from build123d import *

# Parameters (mm, degrees)
SKETCH_1_W          = 100
SKETCH_1_H          = 80
SKETCH_1_R          = 1.5
SKETCH_1_R_2        = 2.5
EXTRUDE_1_DEPTH     = 3
SKETCH_2_R          = 1.5
CUT_EXTRUDE_1_DEPTH = 10
SKETCH_3_R          = 2
CUT_EXTRUDE_2_DEPTH = 65.101482042


with BuildPart() as part:
    # 草图1 → 凸台-拉伸1 (new body)
    with BuildSketch(Plane.XY):
        Rectangle(SKETCH_1_W, SKETCH_1_H)
        with Locations((0, 14)):
            Circle(SKETCH_1_R, mode=Mode.SUBTRACT)
        with Locations((12.124355653, 7)):
            Circle(SKETCH_1_R, mode=Mode.SUBTRACT)
        with Locations((12.124355653, -7)):
            Circle(SKETCH_1_R, mode=Mode.SUBTRACT)
        with Locations((0, -14)):
            Circle(SKETCH_1_R, mode=Mode.SUBTRACT)
        with Locations((-12.124355653, -7)):
            Circle(SKETCH_1_R, mode=Mode.SUBTRACT)
        with Locations((-12.124355653, 7)):
            Circle(SKETCH_1_R, mode=Mode.SUBTRACT)
        Circle(SKETCH_1_R_2, mode=Mode.SUBTRACT)
    extrude(amount=EXTRUDE_1_DEPTH)

    # 草图2 → 切除-拉伸1 (cut)
    with BuildSketch(Plane(origin=(0, 0, 0), x_dir=(-1, 0, 0), z_dir=(0, 0, -1))):
        with Locations((-40, 35)):
            Circle(SKETCH_2_R)
        with Locations((-30, 35)):
            Circle(SKETCH_2_R)
        with Locations(Location((30, 35, 0), (0, 0, 180))):
            Circle(SKETCH_2_R)
        with Locations(Location((40, 35, 0), (0, 0, 180))):
            Circle(SKETCH_2_R)
        with Locations((40, -35)):
            Circle(SKETCH_2_R)
        with Locations((30, -35)):
            Circle(SKETCH_2_R)
        with Locations(Location((-30, -35, 0), (0, 0, 180))):
            Circle(SKETCH_2_R)
        with Locations(Location((-40, -35, 0), (0, 0, 180))):
            Circle(SKETCH_2_R)
    extrude(amount=-CUT_EXTRUDE_1_DEPTH, mode=Mode.SUBTRACT)

    # 草图3 → 切除-拉伸2 (cut, through all)
    with BuildSketch(Plane(origin=(0, 0, 0), x_dir=(-1, 0, 0), z_dir=(0, 0, -1))):
        with Locations((34.641016151, 20)):
            Circle(SKETCH_3_R)
    extrude(amount=-CUT_EXTRUDE_2_DEPTH, mode=Mode.SUBTRACT)


solid = part.part
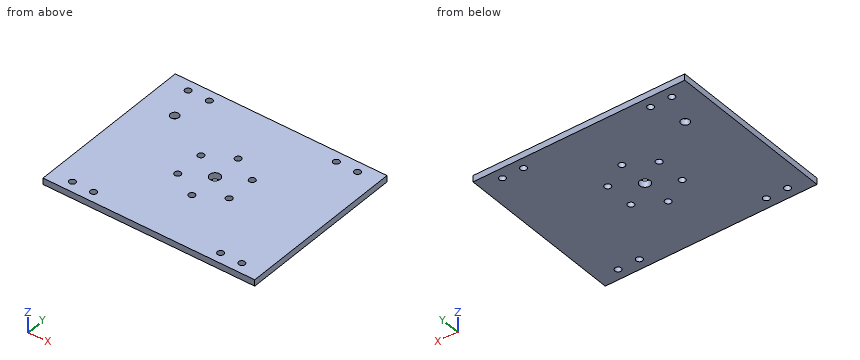
The listing builds one solid part. Answer for the finished solid, in the listing's coordinates (mm). Give positions to 0.01 mm unless a question says otherwise; leave off trailing zeros. Loops run counter-clockwise (first coordinate to the right, second up) from the corner with the lowest first, then second, coordinate; pieces in that order, holes last. Notation, with made-up numbers: (-36.5, 72) - (-25.5, 72) arc R14 cw to (-25.5, 84) - close; hole circle Ø1 at (9.5, -25.75). An arc over 180 degrees is marked (long way). Write each question's results on one line, items separated by ' | '.
1. Find section A-A, the plane y = -14. Write down the section's boundary in (x, z), then the cut area to 3 significant figures.
Resolved:
outline: (-50, 0) - (-1.5, 0) - (-1.5, 3) - (-50, 3) - close; (1.5, 0) - (50, 0) - (50, 3) - (1.5, 3) - close | area: 291 mm^2
2. Consider probe 1 along Y at (x, z) = (30, 1.25). Determine where the line is inside the solid, lowest interval first. Write a range as from..to.
Resolved:
probe 1: y = -40..-36.5, -33.5..33.5, 36.5..40
3. Find section D-D, the plane x = -30. Write down the section's boundary in (y, z).
Resolved:
outline: (-40, 0) - (-36.5, 0) - (-36.5, 3) - (-40, 3) - close; (-33.5, 0) - (33.5, 0) - (33.5, 3) - (-33.5, 3) - close; (36.5, 0) - (40, 0) - (40, 3) - (36.5, 3) - close
4. Find section C-C, the plane z = 2.2. Count the separate pieces of the cut face and the enclosed holes in it, then the cut area to 3 significant figures.
Resolved:
separate pieces: 1 | enclosed holes: 16 | area: 7,870 mm^2
5. Find section B-B, the plane y = -35. Write down the section's boundary in (x, z).
Resolved:
outline: (-50, 0) - (-41.5, 0) - (-41.5, 3) - (-50, 3) - close; (-38.5, 0) - (-31.5, 0) - (-31.5, 3) - (-38.5, 3) - close; (-28.5, 0) - (28.5, 0) - (28.5, 3) - (-28.5, 3) - close; (31.5, 0) - (38.5, 0) - (38.5, 3) - (31.5, 3) - close; (41.5, 0) - (50, 0) - (50, 3) - (41.5, 3) - close
6. A flat-ended cylindrical pin translates along its axis: P1, Ø2.5, axis at x = -30, y = -35, coming from the +Z side. Find the tip coordinate at first contact, or state that the pin passes through.
Resolved:
P1: passes through
